```python
from build123d import *

# Parameters (mm, degrees)
F1_DEPTH = 15
F2_R     = 3
F3_DEPTH = 15.001
F4_R     = 3
F5_DEPTH = 10


with BuildPart() as f1:
    # F0 (on Top) → F1 (new body)
    with BuildSketch(Plane.XY):
        with BuildLine():
            ThreePointArc((9.3561974046, -1.7852717232), (9.4827054494, -0.8966171761), (9.525, 0))
            ThreePointArc((9.525, 0), (9.4827054494, 0.8966171761), (9.3561974046, 1.7852717232))
            ThreePointArc((9.3561974046, 1.7852717232), (7.9216471704, 2.5738991923), (8.6186790933, 4.0551196883))
            ThreePointArc((8.6186790933, 4.0551196883), (7.7058868714, 5.5986545281), (6.5199663128, 6.9437500156))
            ThreePointArc((6.5199663128, 6.9437500156), (4.8958471982, 6.738555569), (4.5891183065, 8.3465932074))
            ThreePointArc((4.5891183065, 8.3465932074), (2.9433868714, 9.0588133177), (1.193329695, 9.4499518115))
            ThreePointArc((1.193329695, 9.4499518115), (0, 8.3293127534), (-1.193329695, 9.4499518115))
            ThreePointArc((-1.193329695, 9.4499518115), (-2.9433868714, 9.0588133177), (-4.5891183065, 8.3465932074))
            ThreePointArc((-4.5891183065, 8.3465932074), (-4.4504477573, 8.039487236), (-4.4029672815, 7.7058868714))
            ThreePointArc((-4.4029672815, 7.7058868714), (-5.1936438859, 6.5808827064), (-6.5199663128, 6.9437500156))
            ThreePointArc((-6.5199663128, 6.9437500156), (-7.7058868714, 5.5986545281), (-8.6186790933, 4.0551196883))
            ThreePointArc((-8.6186790933, 4.0551196883), (-8.0698919683, 3.6154750772), (-7.8631260711, 2.9433868714))
            ThreePointArc((-7.8631260711, 2.9433868714), (-8.3259799016, 1.9985995007), (-9.3561974046, 1.7852717232))
            ThreePointArc((-9.3561974046, 1.7852717232), (-9.525, 0), (-9.3561974046, -1.7852717232))
            ThreePointArc((-9.3561974046, -1.7852717232), (-8.3259799016, -1.9985995007), (-7.8631260711, -2.9433868714))
            ThreePointArc((-7.8631260711, -2.9433868714), (-8.0698919683, -3.6154750772), (-8.6186790933, -4.0551196883))
            ThreePointArc((-8.6186790933, -4.0551196883), (-7.7058868714, -5.5986545281), (-6.5199663128, -6.9437500156))
            ThreePointArc((-6.5199663128, -6.9437500156), (-5.1936438859, -6.5808827064), (-4.4029672815, -7.7058868714))
            ThreePointArc((-4.4029672815, -7.7058868714), (-4.4504477573, -8.039487236), (-4.5891183065, -8.3465932074))
            ThreePointArc((-4.5891183065, -8.3465932074), (-2.9433868714, -9.0588133177), (-1.193329695, -9.4499518115))
            ThreePointArc((-1.193329695, -9.4499518115), (0, -8.3293127534), (1.193329695, -9.4499518115))
            ThreePointArc((1.193329695, -9.4499518115), (2.9433868714, -9.0588133177), (4.5891183065, -8.3465932074))
            ThreePointArc((4.5891183065, -8.3465932074), (4.8958471982, -6.738555569), (6.5199663128, -6.9437500156))
            ThreePointArc((6.5199663128, -6.9437500156), (7.7058868714, -5.5986545281), (8.6186790933, -4.0551196883))
            ThreePointArc((8.6186790933, -4.0551196883), (7.9216471704, -2.5738991923), (9.3561974046, -1.7852717232))
        make_face()
    extrude(amount=F1_DEPTH)

    # F2 (on face) → F3 (cut, through all)
    with BuildSketch(Plane.XY.offset(15)):
        Circle(F2_R)
    extrude(amount=-F3_DEPTH, mode=Mode.SUBTRACT)

    # F4 (on face) → F5 (cut)
    with BuildSketch(Plane.XY.offset(15)):
        Polygon((2.8867513459, -5), (5.7735026919, 0), (2.8867513459, 5), (-2.8867513459, 5), (-5.7735026919, 0), (-2.8867513459, -5), align=None)
        Circle(F4_R, mode=Mode.SUBTRACT)
    extrude(amount=-F5_DEPTH, mode=Mode.SUBTRACT)


solid = f1.part
```
Input: part model. Units: mm. Frame: model coordinates. A direction names the side the tool comes from. Round coordinates to 2 decimals unless told otherwise and drop trailing zeros. Loops run counter-clockwise (first coordinate to the right, second up) from the corner with the lowest first, then second, coordinate; pieces in that order, holes last. Notation, with made-up numbers: (-21.5, 63) -> (-6.5, 63) arc R11 ccw to (-6.5, 69) -> close; hole circle Ø7 at (45.5, -32). An arc over 180 degrees is marked (long way). Use one line per item in the form item = value. Start each with the question number.
Item 1: Section query D-D on x = -3.5. Return the cut outline in (y, z), then the cut area to 3 significant figures.
Item 2: Material intervals for L1, parallel to Y at x = 0, z = 1.15; L2, parallel to Y at x = -5, z = 7; L3, parallel to X at y = -8.5, z = 9.5, sorted ascending. Write a range as from..to.
Item 3: Section query C-C on y = 0.5. Return the cut outline in (x, z).
Item 4: Set-up query: faces 1 (the face through (-4.31, 2.535, 10.07)), 2 (the face through (7.93, 2.55, 7.4)). Return all of +Z, -Z, +X, -X, +Y, -Y with unobstructed straight access to the full face (end or side cutting, diameter ignored); none if empty.
Item 5: Mould query, pull axis X, two halves, no side actions, for faces 3 (the face through (4.31, -2.535, 10.07)), 4 (the face through (2.919, -9.067, 7.395)), 5 (the face through (-2.919, 9.067, 7.395)). Classes: pulls with the +X half, pulls with the -X half, needs draft (parallel to the pull), parting line crosses it, or undercut.
Item 6: Section query A-A on x = 0. Return the cut outline in (y, z), then the cut area to 3 significant figures.
Item 7: Contact query for flat-ended pins moving along their axis: pin 1 Ø3 at (x, y) = (0, 0) entering from +Z; pin 2 Ø2 at (x, z) = (-4, 6.5) entering from +Y; pin 3 Ø1 at (y, z) = (-6.5, 2.5) entering from -X; pin 4 Ø5 at (x, z) = (-5.5, 12.5) entering from -Y. Output: stop coordinate, or through.
Ans:
q1.outline = (-8.86, 0) -> (8.86, 0) -> (8.86, 15) -> (3.94, 15) -> (3.94, 5) -> (-3.94, 5) -> (-3.94, 15) -> (-8.86, 15) -> close
q1.area = 187 mm^2
q2.L1 = -8.33..-3, 3..8.33
q2.L2 = -6.67..-1.34, 1.34..6.67
q2.L3 = -4.3..-0.62, 0.62..4.3
q3.outline = (-9.51, 0) -> (-2.96, 0) -> (-2.96, 5) -> (-5.48, 5) -> (-5.48, 15) -> (-9.51, 15) -> close; (2.96, 0) -> (9.51, 0) -> (9.51, 15) -> (5.48, 15) -> (5.48, 5) -> (2.96, 5) -> close
q4.face_1 = +Z
q4.face_2 = +Z, -Z
q5.face_3 = undercut
q5.face_4 = pulls with the +X half
q5.face_5 = pulls with the -X half
q6.outline = (-8.33, 0) -> (-3, 0) -> (-3, 5) -> (-5, 5) -> (-5, 15) -> (-8.33, 15) -> close; (3, 0) -> (8.33, 0) -> (8.33, 15) -> (5, 15) -> (5, 5) -> (3, 5) -> close
q6.area = 120 mm^2
q7.pin_1 = through
q7.pin_2 = 9.04
q7.pin_3 = -7.4
q7.pin_4 = -9.04
